Autodesk Fusion 360 part; units mm, degrees
sketch "スケッチ1" plane through (0, 0, 0) normal (0, 0, 1) x (1, 0, 0)
  line L0 (9, 120.8679) -> (9, 29.1321)
  line L1 (0, 150) -> (0, 0)
  line L2 (0, 0) -> (75, 0)
  line L3 (22.6927, 14.1892) -> (75, 9.6129)
  arc A0 (9, 29.1321) -> (22.6927, 14.1892) centre (24, 29.1321) ccw
  line L4 (75, 9.6129) -> (75, 0)
  line L5 (75, 140.3871) -> (22.6927, 135.8108)
  line L6 (0, 150) -> (75, 150)
  arc A1 (22.6927, 135.8108) -> (9, 120.8679) centre (24, 120.8679) ccw
  line L7 (75, 150) -> (75, 140.3871)
extrude "押し出し1" add sketch "スケッチ1" along normal blind 100
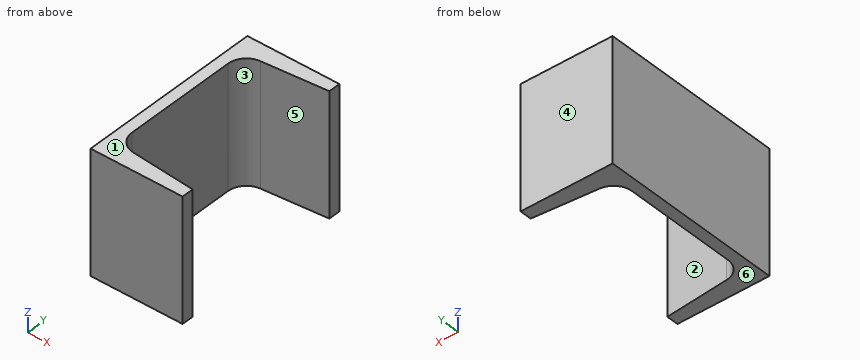
Verification items for the finished model (mm, model axes). Face numbers are marked on the shaded views. A direction names the side the tool comes from. Coordinates: 2 decimals unless noted, no trailing zeros. Write each loop counter-clockwise with the first axis right and the second up, starting at its lowest first coordinate (ties: lowest second). Pieces come first, ordered by that corner, then holes. Notation, with made-up numbers: (20.5, 66.25) - (55.5, 66.25) arc R21 cw to (55.5, 84.25) - close; hole circle Ø6 at (0.25, 78). An arc over 180 degrees is marked (long way). One line per question, with ' | ' between items. Start each with the question number.
1. Section check A-A (z = 12.5). Enter the section's corners in (x, y).
2. Access from +Z, -Z, +X, -X, +Y, -Y to the whole of each face (thin tool, end or side, straight path). Record for the marked faces 1 and 2.
3. Draft check along Y on the marked faces 3, 4, 5 and 6. Enter one of: released by +Y, released by -Y, zero draft, split by the parting line, or undercut.
4. Section check D-D (x = 16.5). Enter the section's corners in (y, z).
5. Material ranges on line 1 along X through (y, z) = (104, 50.5); line 2 along Y through (x, z) = (33.5, 14.5); line 3 along Y through (x, z) = (19, 47.5), recorded low to high.
6. Gauge pin test, flat ends, axial feed: P1, Ø8, axis at y = 51.5, z = 34.5, coming from the +X side; P2, Ø10, axis at y = 23.5, z = 38, coming from the +X side. Record the tip position at first contact, or that the pin passes through.
7. Section check C-C (y = 84). Enter the section's corners in (x, z).
8. Section check B-B (x = 24.5). Enter the section's corners in (y, z), plus the area to 3 significant figures.
Computed values:
1) outline: (0, 0) - (75, 0) - (75, 9.61) - (22.69, 14.19) arc R15 cw to (9, 29.13) - (9, 120.87) arc R15 cw to (22.69, 135.81) - (75, 140.39) - (75, 150) - (0, 150) - close
2) face 1: +Z, +X, -X, +Y, -Y | face 2: +Z, -Z, +X
3) face 3: undercut | face 4: released by +Y | face 5: undercut | face 6: zero draft
4) outline: (0, 0) - (16.14, 0) - (16.14, 100) - (0, 100) - close; (133.86, 0) - (150, 0) - (150, 100) - (133.86, 100) - close
5) line 1: 0 to 9 | line 2: 0 to 13.24, 136.76 to 150 | line 3: 0 to 14.99, 135.01 to 150
6) P1: x = 9 | P2: x = 13.42
7) outline: (0, 0) - (9, 0) - (9, 100) - (0, 100) - close
8) outline: (0, 0) - (14.03, 0) - (14.03, 100) - (0, 100) - close; (135.97, 0) - (150, 0) - (150, 100) - (135.97, 100) - close | area: 2,810 mm²
